```python
from build123d import *

# Parameters (mm, degrees)
F1_DEPTH = 9
F2_R     = 4


with BuildPart() as f1:
    # F0 (on Front) → F1 (new body)
    with BuildSketch(Plane.XZ):
        with BuildLine():
            Line((-10, 8), (-10, 0))
            Line((-10, 0), (0, 0))
            Line((0, 0), (0, 18))
            ThreePointArc((0, 18), (-7.071068, 15.071068), (-10, 8))
        make_face()
    extrude(amount=F1_DEPTH)

    # F2
    f2_edges = [f1.edges().sort_by_distance(p)[0] for p in [
        (-7.071068, 0, 15.071068),
        (-10, 0, 4),
        (-10, -9, 4),
        (-7.071068, -9, 15.071068),
    ]]
    fillet(f2_edges, radius=F2_R)


solid = f1.part
```
Geometry: final body of the model. Coordinates: model frame, mm. Give positions to 0.01 mm unless a question says otherwise; leave off trailing zeros. Loops run counter-clockwise (first coordinate to the right, second up) from the corner with the lowest first, then second, coordinate; pieces in that order, holes last. Notation, with made-up numbers: (76, 50) -> (105, 50) arc R13 ccw to (105, 61) -> close; hole circle Ø6 at (52.5, 1.25). An arc over 180 degrees is marked (long way). Use CSV: the item, a comma, the result in double quotes.
(1) Cut plane C-C (y = -2.25). Output: boundary loops of the cut face in (x, z), plus the area to 3 significant figures.
From the geometry:
outline,"(-9.6, 0) -> (0, 0) -> (0, 17.6) arc R9.6 ccw to (-9.6, 8) -> close"
area,"149 mm^2"
(2) Cut plane A-A (z = 7). Output: boundary loops of the cut face in (x, y), plus the area to 3 significant figures.
From the geometry:
outline,"(-10, -5) arc R4 ccw to (-6, -9) -> (0, -9) -> (0, 0) -> (-6, 0) arc R4 ccw to (-10, -4) -> close"
area,"83.1 mm^2"
(3) Ray query, line 1 along Y through (x, z) = (-2.75, 13.5); line 2 along Z through (x, y) = (-3, -5.5); line 3 along Z through (x, y) = (-2.75, -0.5). Return the intervals inside material, ascending. Write a range as [from, to].
From the geometry:
line 1,"[-9, 0]"
line 2,"[0, 17.51]"
line 3,"[0, 15.44]"
(4) Cut plane B-B (y = -4.75). Output: boundary loops of the cut face in (x, z).
From the geometry:
outline,"(-10, 0) -> (0, 0) -> (0, 18) arc R10 ccw to (-10, 8) -> close"
(5) First-contact query: P1, Ø5, axis at x = -3.5, y = -5.5, coming from the +Z side; P2, Ø4, axis at x = -7, z = 15, coming from the -Y side; P3, Ø2, axis at x = -4.5, y = -6.5, coming from the +Z side. Flat tips, straight axial feed; report the tip coordinate or a pass-through.
From the geometry:
P1,"z = 17.95"
P2,"y = -8.52"
P3,"z = 17.18"
